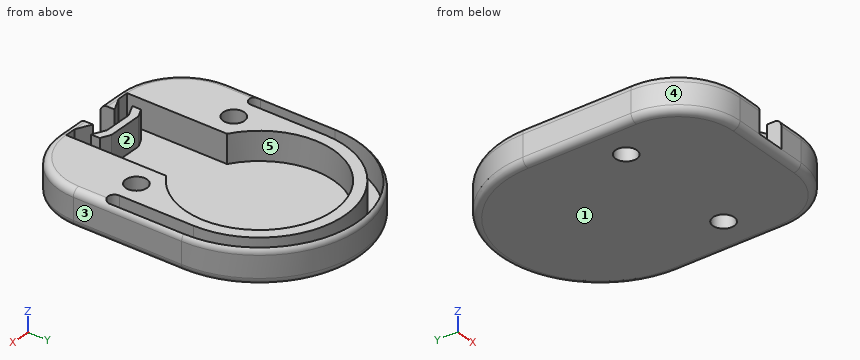
```python
from build123d import *

# Parameters (mm, degrees)
PAD020_DEPTH         = 2
PAD020_DEPTH_BACK    = 0.5
FILLET003_R          = 0.49
POCKET007_DEPTH      = 2.001
SKETCH044_R          = 0.75
POCKET008_DEPTH      = 2.0010001
POCKET008_DEPTH_BACK = 0.501


with BuildPart() as part:
    # Sketch040 → Pad020 (new body, two sides)
    with BuildSketch(Plane.XY) as pad020_sk:
        with BuildLine():
            ThreePointArc((7.15, 0), (0, 7.15), (-7.15, 0))
            Line((-7.15, 0), (-7.15, -7.65))
            ThreePointArc((-7.15, -7.65), (-5.8759144982, -10.7259144982), (-2.8, -12))
            Line((-2.8, -12), (2.8, -12))
            ThreePointArc((2.8, -12), (5.8759144982, -10.7259144982), (7.15, -7.65))
            Line((7.15, 0), (7.15, -7.65))
        make_face()
    extrude(amount=PAD020_DEPTH)
    extrude(pad020_sk.sketch, amount=-PAD020_DEPTH_BACK)

    # Fillet003
    fillet003_edges = [part.edges().sort_by_distance(p)[0] for p in [
        (0, 7.15, -0.5),
        (-7.15, -3.825, -0.5),
        (-5.875914, -10.725914, -0.5),
        (0, -12, -0.5),
        (5.875914, -10.725914, -0.5),
        (7.15, -3.825, -0.5),
        (0, 7.15, 2),
        (-7.15, -3.825, 2),
        (-5.875914, -10.725914, 2),
        (0, -12, 2),
        (5.875914, -10.725914, 2),
        (7.15, -3.825, 2),
    ]]
    fillet(fillet003_edges, radius=FILLET003_R)

    # Sketch043 → Pocket007 (cut, through all)
    with BuildSketch(Plane.XY):
        with BuildLine():
            Line((1, -12), (1, -11))
            Line((1, -11), (2.0323708024, -11.5))
            Line((2.0323708024, -11.5), (2.8, -11.5))
            Line((2.8, -11.5), (2.8, -4.4410021392))
            ThreePointArc((2.8, -4.4410021392), (0, 5.25), (-2.8, -4.4410021392))
            Line((-2.8, -11.5), (-2.8, -4.4410021392))
            Line((-2.8, -11.5), (-2.0323708024, -11.5))
            Line((-2.0323708024, -11.5), (-1, -11))
            Line((-1, -11), (-1, -12))
            Line((-1, -12), (1, -12))
        make_face()
        Polygon((1.2421610524, -9.5), (-1.2421610524, -9.5), (-1.9, -9.8186059437), (-1.9, -10.4358898944), (-1, -10), (1, -10), (1.9, -10.4358898944), (1.9, -9.8186059437), align=None, mode=Mode.SUBTRACT)
        with BuildLine():
            ThreePointArc((6.05, 0), (0, 6.05), (-6.05, 0))
            Line((-6.05, -5.25), (-6.05, 0))
            ThreePointArc((-6.95, -5.25), (-6.5, -5.7), (-6.05, -5.25))
            Line((-6.95, 0), (-6.95, -5.25))
            ThreePointArc((6.95, 0), (0, 6.95), (-6.95, 0))
            Line((6.95, 0), (6.95, -5.25))
            ThreePointArc((6.05, -5.25), (6.5, -5.7), (6.95, -5.25))
            Line((6.05, 0), (6.05, -5.25))
        make_face()
    extrude(amount=POCKET007_DEPTH, mode=Mode.SUBTRACT)

    # Sketch044 → Pocket008 (cut, two sides)
    with BuildSketch(Plane.XY) as pocket008_sk:
        with Locations((4.475757, -5.25)):
            Circle(SKETCH044_R)
        with Locations((-4.475757, -5.25)):
            Circle(SKETCH044_R)
    extrude(amount=POCKET008_DEPTH, mode=Mode.SUBTRACT)
    extrude(pocket008_sk.sketch, amount=-POCKET008_DEPTH_BACK, mode=Mode.SUBTRACT)


solid = part.part
```
The model under review builds one solid part; all positions refer to its coordinate system, in mm. Face numbers are marked on the shaded views. A direction names the side the tool comes from. Round coordinates to 2 decimals unless told otherwise and drop trailing zeros. Loops run counter-clockwise (first coordinate to the right, second up) from the corner with the lowest first, then second, coordinate; pieces in that order, holes last. Notation, with made-up numbers: (-21, 35.25) - (32, 35.25) arc R6 ccw to (32, 41.25) - close; hole circle Ø5 at (77.5, 30.25). An arc over 180 degrees is marked (long way). Write each question's results on one line, items separated by ' | '. Start each with the question number.
Q1. Draft analysis for pull direction Y (two halves, no side actions). For the marked faces 3, 4 and 5, state which applies: pulls with the +Y half, pulls with the -Y half, needs draft (parallel to the pull), parting line crosses it, or undercut.
Q2. Take a section at C-C on y = -6.5. Give the boundary of the cut face in (x, z).
Q3. Take a section at A-A on z = 0.6. Give the number of separate pieces and of enclosed holes in the cut face, plus the area to 3 significant figures.
Q4. Wall thickness on line 1 along Y through (x, z) = (0, 1.3); line 2 along Y through (x, z) = (0, 1.95); line 3 along Y through (x, z) = (-4.5, 1.3): over which ranges is each line inside the solid? List them lowest first. Write a range as [from, to].
Q5. Insertion check: P1, Ø1, axis at y = 4, z = 0, coming from the +X side; P2, Ø6.5, axis at x = 0, y = 0, coming from the +Z side; P3, Ø0.8, axis at y = -11.5, z = 1.5, coming from the +X side. Each pin has a flat end and moves straight along its axis. Give the tip position at first contact, or say it passes through.
Q6. Tool access review of the marked faces 1 and 2: name each direction out of +Z, -Z, +X, -X, +Y, -Y from which nothing blocks a thin tool from reaching the whole face with its end or side.
Data:
1) face 3: needs draft | face 4: pulls with the -Y half | face 5: undercut
2) outline: (-7.15, -0.01) arc R0.49 ccw to (-6.66, -0.5) - (6.66, -0.5) arc R0.49 ccw to (7.15, -0.01) - (7.15, 1.51) arc R0.49 ccw to (6.66, 2) - (2.8, 2) - (2.8, 0) - (-2.8, 0) - (-2.8, 2) - (-6.66, 2) arc R0.49 ccw to (-7.15, 1.51) - close
3) separate pieces: 2 | enclosed holes: 3 | area: 90.3 mm²
4) line 1: y = [-10, -9.5], [5.25, 6.05], [6.95, 7.15] | line 2: y = [-10, -9.5], [5.25, 6.05] | line 3: y = [-11.65, -6], [-4.5, -2.7], [2.7, 4.04], [5.3, 5.56]
5) P1: stops at x = 6.23 | P2: stops at z = 0 | P3: stops at x = 5.45
6) face 1: -Z, +X, -X, +Y, -Y | face 2: +Z
